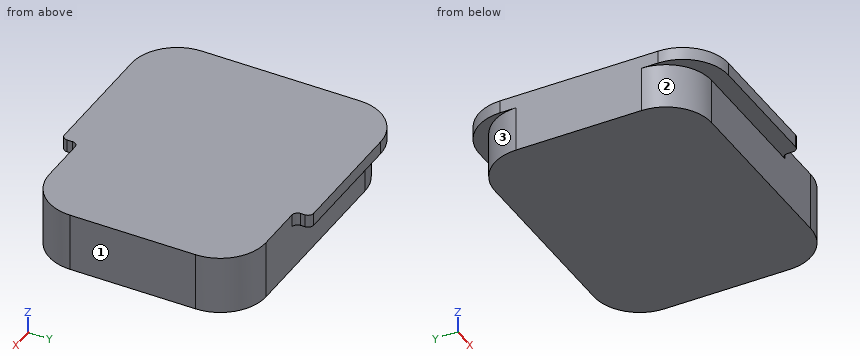
```python
from build123d import *

# Parameters (mm, degrees)
F1_DEPTH = 10.25
F3_DEPTH = 2.25
F4_R     = 1


with BuildPart() as f1:
    # F0 (on Top) → F1 (new body)
    with BuildSketch(Plane.XY):
        with BuildLine():
            Line((16, 19), (-16, 19))
            ThreePointArc((-16, 19), (-21.6568542495, 16.6568542495), (-24, 11))
            Line((-24, 11), (-24, -11))
            ThreePointArc((-24, -11), (-21.6568542495, -16.6568542495), (-16, -19))
            Line((-16, -19), (16, -19))
            ThreePointArc((16, -19), (21.6568542495, -16.6568542495), (24, -11))
            Line((24, -11), (24, 11))
            ThreePointArc((24, 11), (21.6568542495, 16.6568542495), (16, 19))
        make_face()
    extrude(amount=F1_DEPTH)

    # F2 (on face) → F3 (join)
    with BuildSketch(Plane.XY.offset(10.25)):
        with BuildLine():
            Line((6.65, -21.95), (6.65, -19))
            Line((6.65, -19), (-16, -19))
            ThreePointArc((-16, -19), (-21.6568542495, -16.6568542495), (-24, -11))
            Line((-24, -11), (-24, -13.95))
            ThreePointArc((-24, -13.95), (-21.6568542495, -19.6068542495), (-16, -21.95))
            Line((-16, -21.95), (6.65, -21.95))
        make_face()
        with BuildLine():
            Line((6.65, 21.75), (-16, 21.75))
            ThreePointArc((-16, 21.75), (-21.6568542495, 19.4068542495), (-24, 13.75))
            Line((-24, 13.75), (-24, 11))
            ThreePointArc((-24, 11), (-21.6568542495, 16.6568542495), (-16, 19))
            Line((-16, 19), (6.65, 19))
            Line((6.65, 19), (6.65, 21.75))
        make_face()
    extrude(amount=-F3_DEPTH)

    # F4
    f4_edges = [f1.edges().sort_by_distance(p)[0] for p in [
        (6.65, 21.75, 9.125),
        (6.65, -21.95, 9.125),
        (6.65, -19, 9.125),
        (6.65, 19, 9.125),
    ]]
    fillet(f4_edges, radius=F4_R)


solid = f1.part
```
Check sheet for the modelled part. Datum: model origin and axes. Units: mm. Face numbers are marked on the shaded views. A direction names the side the tool comes from. Coordinates: 2 decimals unless noted, no trailing zeros. Order: outer loops, then holes, each group sorted by start corner. A loop starts at its lowest first (then second) coordinate and runs counter-clockwise, first axis right, second up. Notation, with made-up numbers: M -9.75,24 L 4.25,24 A18 cw 4.25,42 Z; hole C -10,-39.75 d3. An arc over 180 degrees is marked long. Write each question's results on one line, items separated by ' | '. Start each with the question number.
1. Cross-section at C-C on y = 15.5. Record the cut outline in (x, z), and give its area (3 significant figures).
2. Cross-section at D-D on x = 13. Record the cut outline in (y, z).
3. Access from +Z, -Z, +X, -X, +Y, -Y to the whole of each face (thin tool, end or side, straight path). Record for the marked faces 1, 2 and 3.
4. Go/stop test with flat-tipped pins: P1, Ø12, axis at x = -10.5, y = 14, coming from the -Z side; P2, Ø1, axis at y = -20.5, z = 9, coming from the +X side; P3, Ø0.6, axis at y = 20.5, z = 9, coming from the +X side; P4, Ø3, axis at y = 15, z = 2, coming from the -X side. Record where each tip stops, or that it passes through.
5. Cross-section at B-B on x = -11.5. Record the cut outline in (y, z).
6. Material ranges on probe 1 along Y at (x, z) = (-2, 1); probe 2 along Y at (x, z) = (-20, 6.25); probe 3 along X at (y, z) = (13, 9.5), recorded low to high.
7. Cross-section at A-A on z = 2.25. Record the cut outline in (x, y).
Checks:
1) outline: M -23.81,8 L -22.61,8 L -22.61,0 L 22.61,0 L 22.61,10.25 L -23.81,10.25 Z | area: 466 mm²
2) outline: M -19,0 L 19,0 L 19,10.25 L -19,10.25 Z
3) face 1: +Z, -Z, +X, +Y, -Y | face 2: -Z, -X, -Y | face 3: -Z, -X, +Y
4) P1: stops at z = 0 | P2: stops at x = 6.65 | P3: stops at x = 6.65 | P4: stops at x = -23.6
5) outline: M -21.95,8 L -19,8 L -19,0 L 19,0 L 19,8 L 21.75,8 L 21.75,10.25 L -21.95,10.25 Z
6) probe 1: y = -19 to 19 | probe 2: y = -17.93 to 17.93 | probe 3: x = -24 to 23.75
7) outline: M -24,-11 A8 ccw -16,-19 L 16,-19 A8 ccw 24,-11 L 24,11 A8 ccw 16,19 L -16,19 A8 ccw -24,11 Z
